Verification items for the finished model (mm, model axes). Round coordinates to 2 decimals unless told otherwise and drop trailing zeros. Loops run counter-clockwise (first coordinate to the right, second up) from the corner with the lowest first, then second, coordinate; pieces in that order, holes last. Notation, with made-up numbers: (61, 53.5) - (82, 53.5) arc R20 cw to (82, 70.5) - close; hole circle Ø7 at (63, -4). An arc over 180 degrees is marked (long way). Use a Markdown table: item, result. Add a question column.
```python
from build123d import *

# Parameters (mm, degrees)
SKETCH1_W           = 500
SKETCH1_H           = 106.02
BOSS_EXTRUDE1_DEPTH = 12
SKETCH2_W           = 12
SKETCH2_H           = 24
CUT_EXTRUDE1_DEPTH  = 512.257508894
SKETCH3_W           = 154.666666667
SKETCH3_H           = 12
CUT_EXTRUDE2_DEPTH  = 512.257508894
SCALE1_SCALE        = 0.5


with BuildPart() as part:
    # Sketch1 → Boss-Extrude1 (new body)
    with BuildSketch(Plane.XY):
        with Locations((250, 53.01)):
            Rectangle(SKETCH1_W, SKETCH1_H)
    extrude(amount=BOSS_EXTRUDE1_DEPTH)

    # Sketch2 → Cut-Extrude1 (cut, through all)
    with BuildSketch(Plane.XY.offset(12)):
        with Locations((494, 12)):
            Rectangle(SKETCH2_W, SKETCH2_H)
        with Locations((494, 94.02)):
            Rectangle(SKETCH2_W, SKETCH2_H)
        with Locations((6, 94.02)):
            Rectangle(SKETCH2_W, SKETCH2_H)
        with Locations((6, 12)):
            Rectangle(SKETCH2_W, SKETCH2_H)
    extrude(amount=-CUT_EXTRUDE1_DEPTH, mode=Mode.SUBTRACT)

    # Sketch3 → Cut-Extrude2 (cut, through all)
    with BuildSketch(Plane.XY.offset(12)):
        with Locations((89.333333334, 6)):
            Rectangle(SKETCH3_W, SKETCH3_H)
        with Locations((410.666666667, 6)):
            Rectangle(SKETCH3_W, SKETCH3_H)
        with Locations((89.333333334, 100.02)):
            Rectangle(SKETCH3_W, SKETCH3_H)
        with Locations((410.666666667, 100.02)):
            Rectangle(SKETCH3_W, SKETCH3_H)
    extrude(amount=-CUT_EXTRUDE2_DEPTH, mode=Mode.SUBTRACT)


with BuildPart() as part_1:
    # Scale1: scaled about (250, 53.01, 6)
    add(part.part.scale(SCALE1_SCALE).moved(Location((125, 26.505, 3))))


solid = part_1.part
```
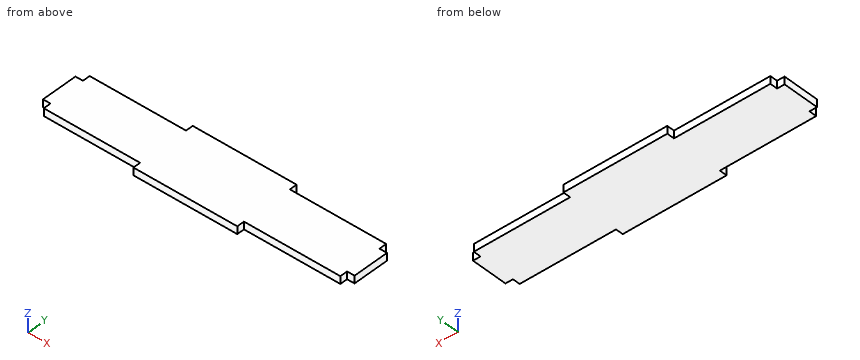
Q1. Section check B-B on x = 201. Record the cut outline in (y, z) (3 decimals).
Q2. Thickness scan on line 1 along Y through (x, z) = (207, 6.4) (3 decimals); line 2 along X through (y, z) = (72, 5.85); line 3 along X through (y, z) = (76.5, 6.35). Record the ranges inside material, lowest first.
Q3. Section check A-A on z = 6.15. Record the cut outline in (x, y) (3 decimals).
Q4. Go/stop test with flat-tipped pins: pin 1 Ø1.5 at (y, z) = (70.5, 7.5) entering from -X; pin 2 Ø1.5 at (y, z) = (72.5, 6) entering from +X; pin 3 Ø1.8 at (y, z) = (28, 6.5) entering from -X. Record where each tip stops, or that it passes through.
Determined:
| question | item | result |
|---|---|---|
| 1 | outline | (32.505, 3) - (73.515, 3) - (73.515, 9) - (32.505, 9) - close |
| 2 | line 1 | y = 32.505 to 73.515 |
| 2 | line 2 | x = 131 to 369 |
| 2 | line 3 | x = 208.33 to 291.67 |
| 3 | outline | (125, 38.505) - (131, 38.505) - (131, 32.505) - (208.333, 32.505) - (208.333, 26.505) - (291.667, 26.505) - (291.667, 32.505) - (369, 32.505) - (369, 38.505) - (375, 38.505) - (375, 67.515) - (369, 67.515) - (369, 73.515) - (291.667, 73.515) - (291.667, 79.515) - (208.333, 79.515) - (208.333, 73.515) - (131, 73.515) - (131, 67.515) - (125, 67.515) - close |
| 4 | pin 1 | stops at x = 131 |
| 4 | pin 2 | stops at x = 369 |
| 4 | pin 3 | stops at x = 208.33 |
